Verification items for this drawing (mm, ordinates from the low corner). A direction names the side the tool comes from. Coordinates: 2 decimals unless noted, no trailing zeros. Loops run counter-clockwise (first coordinate to the right, second up) from the corner with the lowest first, then second, coordinate; pieces in that order, holes last. Notation, with made-up numbers: M 53.25,37 L 68.25,37 A13 ccw 68.25,61 Z; hole C -9.75,76 d6. An arc over 180 degrees is marked long. Return JSON: item names as keys, results as strings.
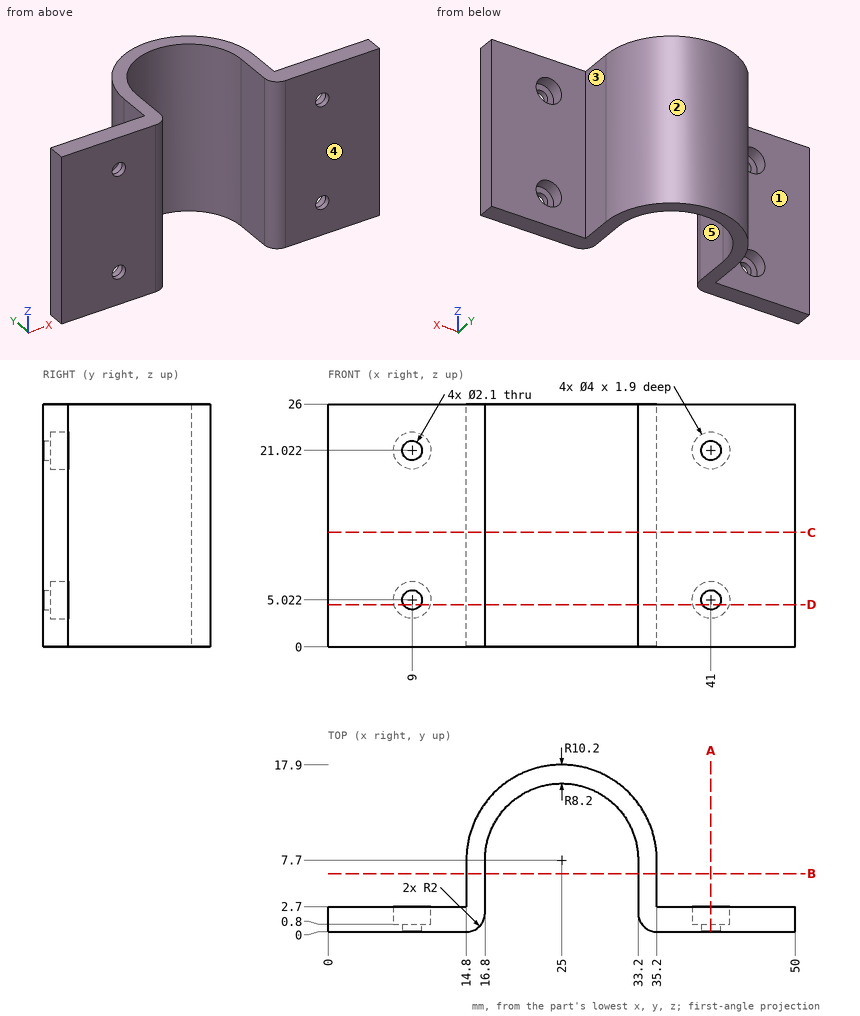
1) Set-up check for the marked faces 1, 2, 3, 4 and 5: record each of +Z, -Z, +X, -X, +Y, -Y from which the full face is reachable in a straight line by a thin tool's end or side.
Answers:
{"face 1": "+Z, -Z, -X, +Y", "face 2": "+Z, -Z, +Y", "face 3": "+Z, -Z, +X, +Y", "face 4": "+Z, -Z, +X, -X, -Y", "face 5": "+Z, -Z, -Y"}
2) Go/stop test with flat-tipped pins: pin 1 Ø2.5 at (x, z) = (41, 21.02) entering from +Y; pin 2 Ø4.5 at (x, z) = (9.5, 6) entering from +Y; pin 3 Ø3 at (y, z) = (14, 9) entering from +X; pin 4 Ø5 at (x, y) = (20.5, 12) entering from -Z. Record where each tip stops, or that it passes through.
Answers:
{"pin 1": "y = 0.8", "pin 2": "y = 2.7", "pin 3": "x = 34", "pin 4": "z = 0"}
3) Section check C-C on z = 12.25. Record the cut outline in (x, y).
Answers:
{"outline": "M 0,0 L 14.8,0 A2 ccw 16.8,2 L 16.8,7.7 A8.2 cw 33.2,7.7 L 33.2,2 A2 ccw 35.2,0 L 50,0 L 50,2.7 L 35.2,2.7 L 35.2,7.7 A10.2 ccw 14.8,7.7 L 14.8,2.7 L 0,2.7 Z"}
4) Scan lines: line 1 along Z through (x, y) = (9, 0.5); line 2 along Z through (x, y) = (9, 1.3); line 3 along X through (y, z) = (6, 15.25). Record each from-to range of solid material in increasing order. Write a range as [from, to].
Answers:
{"line 1": "[0, 3.97], [6.07, 19.97], [22.07, 26]", "line 2": "[0, 3.02], [7.02, 19.02], [23.02, 26]", "line 3": "[14.8, 16.8], [33.2, 35.2]"}
5) Section check B-B on y = 6.25. Record the cut outline in (x, z), then the cut area to 3 significant figures.
Answers:
{"outline": "M 14.8,0 L 16.8,0 L 16.8,26 L 14.8,26 Z; M 33.2,0 L 35.2,0 L 35.2,26 L 33.2,26 Z", "area": "104 mm²"}
6) Section check D-D on z = 4.5. Count the separate pieces of the cut face and the enclosed holes in it, then the cut area to 3 significant figures.
Answers:
{"separate pieces": "3", "enclosed holes": "0", "area": "149 mm²"}
7) Section check A-A on x = 41. Record the cut outline in (y, z).
Answers:
{"outline": "M 0,0 L 2.7,0 L 2.7,3.02 L 0.8,3.02 L 0.8,3.97 L 0,3.97 Z; M 0,6.07 L 0.8,6.07 L 0.8,7.02 L 2.7,7.02 L 2.7,19.02 L 0.8,19.02 L 0.8,19.97 L 0,19.97 Z; M 0,22.07 L 0.8,22.07 L 0.8,23.02 L 2.7,23.02 L 2.7,26 L 0,26 Z"}
